```python
from build123d import *

# Parameters (mm, degrees)
BOSS_EXTRUDE1_DEPTH      = 75
BOSS_EXTRUDE1_DEPTH_BACK = 75
SKETCH1_W                = 40
SKETCH1_H                = 30
SKETCH3_R                = 3.1
CUT_EXTRUDE1_DEPTH       = 150
CUT_EXTRUDE2_DEPTH       = 150
CUT_EXTRUDE2_DEPTH_BACK  = 150
SKETCH4_W                = 22.5
SKETCH4_H                = 15
SKETCH5_R                = 7.6
CUT_EXTRUDE3_DEPTH       = 16
SKETCH7_W                = 58.590655802
SKETCH7_H                = 20
CUT_EXTRUDE5_DEPTH       = 40
SKETCH8_W                = 20
SKETCH8_H                = 35
CUT_EXTRUDE6_DEPTH       = 35
FILLET2_R                = 0.5
FILLET3_R                = 0.5
SKETCH10_R               = 12.5
BOSS_EXTRUDE3_DEPTH      = 15
SKETCH11_W               = 13
SKETCH11_H               = 11
CUT_EXTRUDE7_DEPTH       = 25


with BuildPart() as part:
    # Sketch1 → Boss-Extrude1 (new, two sides: drawn at the far end of the back side and taken through both)
    with BuildSketch(Plane(origin=(0, 0, 0), x_dir=(1, 0, 0), z_dir=(0, 1, 0)).offset(-BOSS_EXTRUDE1_DEPTH_BACK)):
        Rectangle(SKETCH1_W, SKETCH1_H)
    extrude(amount=BOSS_EXTRUDE1_DEPTH + BOSS_EXTRUDE1_DEPTH_BACK)

    # Sketch3 → Cut-Extrude1 (cut)
    with BuildSketch(Plane(origin=(20, 0, 0), x_dir=(0, 0, -1), z_dir=(1, 0, 0))):
        with Locations((0, 30)):
            Circle(SKETCH3_R)
    cut_extrude1 = extrude(amount=-CUT_EXTRUDE1_DEPTH, mode=Mode.SUBTRACT)

    # Mirror1: Cut-Extrude1 across plane
    add(cut_extrude1.mirror(Plane.ZX), mode=Mode.SUBTRACT)

    # Sketch4 → Cut-Extrude2 (cut, two sides: drawn at the far end of the back side and taken through both)
    with BuildSketch(Plane(origin=(0, 0, 0), x_dir=(0, 0, -1), z_dir=(1, 0, 0)).offset(-CUT_EXTRUDE2_DEPTH_BACK)):
        Rectangle(SKETCH4_W, SKETCH4_H)
    extrude(amount=CUT_EXTRUDE2_DEPTH + CUT_EXTRUDE2_DEPTH_BACK, mode=Mode.SUBTRACT)

    # Sketch5 → Cut-Extrude3 (cut)
    with BuildSketch(Plane(origin=(0, 0, -15), x_dir=(-1, 0, 0), z_dir=(0, 0, -1))):
        Circle(SKETCH5_R)
    extrude(amount=-CUT_EXTRUDE3_DEPTH, mode=Mode.SUBTRACT)

    # Sketch7 → Cut-Extrude5 (cut)
    with BuildSketch(Plane(origin=(0, 75, 0), x_dir=(1, 0, 0), z_dir=(0, 1, 0))):
        with Locations((14.295327901, 0)):
            Rectangle(SKETCH7_W, SKETCH7_H)
    extrude(amount=-CUT_EXTRUDE5_DEPTH, mode=Mode.SUBTRACT)

    # Sketch8 → Cut-Extrude6 (cut)
    with BuildSketch(Plane(origin=(20, 0, 0), x_dir=(0, 0, -1), z_dir=(1, 0, 0))):
        with Locations((0, -52.5)):
            Rectangle(SKETCH8_W, SKETCH8_H)
    extrude(amount=-CUT_EXTRUDE6_DEPTH, mode=Mode.SUBTRACT)

    # Fillet2
    fillet2_edges = [part.edges().sort_by_distance(p)[0] for p in [
        (20, 75, 12.5),
        (0, 75, -15),
        (-20, 75, 0),
        (0, 75, 15),
        (20, 75, -12.5),
        (2.5, 75, -10),
        (2.5, 75, 10),
        (-15, 75, 0),
    ]]
    fillet(fillet2_edges, radius=FILLET2_R)

    # Fillet3
    fillet3_edges = [part.edges().sort_by_distance(p)[0] for p in [
        (20, -52.5, 10),
        (20, -70, 0),
        (20, -52.5, -10),
        (20, -35, 0),
    ]]
    fillet(fillet3_edges, radius=FILLET3_R)

    # Sketch10 → Boss-Extrude3 (add)
    with BuildSketch(Plane.XY.offset(15)):
        Circle(SKETCH10_R)
    extrude(amount=BOSS_EXTRUDE3_DEPTH)

    # Sketch11 → Cut-Extrude7 (cut)
    with BuildSketch(Plane.XY.offset(30)):
        Rectangle(SKETCH11_W, SKETCH11_H)
    extrude(amount=-CUT_EXTRUDE7_DEPTH, mode=Mode.SUBTRACT)


solid = part.part
```
For this review, take the finished solid that the model builds, in its own axes (mm). A direction names the side the tool comes from. Give positions to 0.01 mm unless a question says otherwise; leave off trailing zeros. Write each loop counter-clockwise with the first axis right and the second up, starting at its lowest first coordinate (ties: lowest second). Pieces come first, ordered by that corner, then holes.
Item 1: Wall thickness on probe 1 along Y at (x, z) = (6.5, 0); probe 2 along Y at (x, z) = (0, -9); probe 3 along Y at (x, z) = (16, -8): over which ranges is each line inside the solid? List them lowest first.
Item 2: Take a section at D-D (y = 0). Give the boundary of the cut face in (x, z), and give its area (3 significant figures).
Item 3: Machinability: for faces 1 (the face through (2, -35, 0)), 2 (the face through (0, -7, 11.25)), 3 (the face through (6.5, 0, 21)), 4 (the face through (2, 55, -10)), which of the approach directions +Z, -Z, +X, -X, +Y, -Y give a long, thin tool a straight path to every point of the face, cutting with its end or side? Answer none if there is none.
Item 4: Take a section at B-B (z = 8). Give the boundary of the cut face in (x, y).
Item 5: The part is to be moulded in two halves that separate along X. For faces 5 (the face through (0, 6, 30)), 6 (the face through (-6.5, 0, 21)), 7 (the face through (-15, -52, 0)), 8 (the face through (11.923, 3.755, 22.395)), say which applies: +X half, -X half, draft (parallel to the pull), parting line (faces both ways), or undercut.
Item 6: Take a section at A-A (x = 3.5). Give the number of separate pieces and of enclosed holes in the cut face, and give its area (3 significant figures).
Item 7: Take a section at C-C (y = 30). Give the boundary of the cut face in (x, z), and give its area (3 significant figures).
Item 8: Insertion check: P1, Ø4, axis at x = 0.5, y = -23, coming from the +Z side; P2, Ø14.5, axis at x = 0, z = 22, coming from the +Y side; P3, Ø10, axis at x = 5.5, z = -2, coming from the +Y side; P4, Ø1, axis at y = 24, z = 17, coming from the -X side. Each pin has a flat end and moves straight along its axis. Give the tip position at first contact, or say it passes through.
Established:
1. probe 1: y = -75 to -70, -35 to -33.1, -26.9 to -7.5, 7.5 to 26.9, 33.1 to 35
1. probe 2: y = -75 to -70, -35 to -7.6, 7.6 to 35
1. probe 3: y = -75 to -70, -35 to -7.5, 7.5 to 35
2. outline: (-20, -15) - (-7.6, -15) - (-7.6, -11.25) - (-20, -11.25) - close; (-20, 11.25) - (-6.5, 11.25) - (-6.5, 30) - (-12.5, 30) - (-12.5, 15) - (-20, 15) - close; (6.5, 11.25) - (20, 11.25) - (20, 15) - (12.5, 15) - (12.5, 30) - (6.5, 30) - close; (7.6, -15) - (20, -15) - (20, -11.25) - (7.6, -11.25) - close
2. area: 374 mm2
3. face 1: +X
3. face 2: +X, -X
3. face 3: +Z
3. face 4: +X, +Y
4. outline: (-20, -75) - (20, -75) - (20, -70.5) arc R0.5 ccw to (19.5, -70) - (-15, -70) - (-15, -35) - (19.5, -35) arc R0.5 ccw to (20, -34.5) - (20, -7.5) - (-20, -7.5) - close; (-20, 7.5) - (20, 7.5) - (20, 35) - (-15, 35) - (-15, 74.5) arc R0.5 ccw to (-15.5, 75) - (-19.5, 75) arc R0.5 ccw to (-20, 74.5) - close
5. face 5: draft
5. face 6: undercut
5. face 7: +X half
5. face 8: parting line
6. separate pieces: 2
6. enclosed holes: 3
6. area: 2,710 mm2
7. outline: (-20, -15) - (20, -15) - (20, -3.1) - (-20, -3.1) - close; (-20, 3.1) - (20, 3.1) - (20, 15) - (-20, 15) - close
7. area: 952 mm2
8. P1: stops at z = 15
8. P2: stops at y = 74.93
8. P3: stops at y = 35
8. P4: passes through
